Can you work these out from the model? Positions are in its coordinate system, mm. A direction names the side the tool comes from. Round coordinates to 2 decimals unless told otherwise and drop trailing zeros. Order: outer loops, then holes, each group sorted by start corner. A loop starts at its lowest first (then second) coordinate and runs counter-clockwise, first axis right, second up.
Q1. Will this pin go through, and if not, where does the flat tip stop? P1, Ø1, axis at x = -30, y = 16, coming from the -Z side.
Q2. If we section it at D-D (x = 27): Please give me the cut outline in (y, z), plus the area to 3 significant figures.
Q3. If I drill on line 1 (Y direction, x = -27.5, z = 1.7); line 2 (Y direction, x = 36.5, z = 2.05); line 3 (X direction, y = -19.5, z = 0.45), over which ranges is the centre line in solid material (lowest first)?
Q4. We'd pull the mould along Y, two halves only. Please class faces 1 (the face through (42.5, 0, 2)), 2 (the face through (-1, 30, 2)), 3 (the face through (26, 19, 2)): pulls with the +Y half, pulls with the -Y half, needs draft (parallel to the pull), parting line crosses it, or undercut.
Q5. If we section it at C-C (x = -36.5): Please give me the cut outline in (y, z), plus the area to 3 significant figures.
Q6. If we section it at B-B (z = 0.9): Count the separate pieces of the cut face and the enclosed holes in it, plus the area to 3 significant figures.
Q7. For faces 4 (the face through (-32, -20.75, 2)), 5 (the face through (-1, -30, 2)), which set-ups out of +Z, -Z, +X, -X, +Y, -Y let a thin tool reach every point of the face, with its end or its side?
Q8. If we section it at A-A (y = -24.5): Please give me the cut outline in (x, z).
from build123d import *

# Parameters (mm, degrees)
SKETCH1_W              = 85
SKETCH1_H              = 60
SKETCH1_R              = 1.75
SKETCH1_W_2            = 12
SKETCH1_H_2            = 3.5
ELECTRONICS_DECK_DEPTH = 3.2


with BuildPart() as part:
    # Sketch1 → Electronics deck (new body)
    with BuildSketch(Plane.XY):
        Rectangle(SKETCH1_W, SKETCH1_H)
        with Locations((-36.5, -24.5)):
            Circle(SKETCH1_R, mode=Mode.SUBTRACT)
        with Locations((36.5, -24.5)):
            Circle(SKETCH1_R, mode=Mode.SUBTRACT)
        with Locations((-36.5, 24.5)):
            Circle(SKETCH1_R, mode=Mode.SUBTRACT)
        with Locations((36.5, 24.5)):
            Circle(SKETCH1_R, mode=Mode.SUBTRACT)
        with Locations((-32, 19)):
            Rectangle(SKETCH1_W_2, SKETCH1_H_2, mode=Mode.SUBTRACT)
        with Locations((32, 19)):
            Rectangle(SKETCH1_W_2, SKETCH1_H_2, mode=Mode.SUBTRACT)
        with Locations((-32, -19)):
            Rectangle(SKETCH1_W_2, SKETCH1_H_2, mode=Mode.SUBTRACT)
        with Locations((32, -19)):
            Rectangle(SKETCH1_W_2, SKETCH1_H_2, mode=Mode.SUBTRACT)
    extrude(amount=ELECTRONICS_DECK_DEPTH)


solid = part.part
Solution:
1. P1: stops at z = 0
2. outline: (-30, 0) - (-20.75, 0) - (-20.75, 3.2) - (-30, 3.2) - close; (-17.25, 0) - (17.25, 0) - (17.25, 3.2) - (-17.25, 3.2) - close; (20.75, 0) - (30, 0) - (30, 3.2) - (20.75, 3.2) - close
2. area: 170 mm2
3. line 1: y = -30 to -20.75, -17.25 to 17.25, 20.75 to 30
3. line 2: y = -30 to -26.25, -22.75 to -20.75, -17.25 to 17.25, 20.75 to 22.75, 26.25 to 30
3. line 3: x = -42.5 to -38, -26 to 26, 38 to 42.5
4. face 1: needs draft
4. face 2: pulls with the +Y half
4. face 3: undercut
5. outline: (-30, 0) - (-26.25, 0) - (-26.25, 3.2) - (-30, 3.2) - close; (-22.75, 0) - (-20.75, 0) - (-20.75, 3.2) - (-22.75, 3.2) - close; (-17.25, 0) - (17.25, 0) - (17.25, 3.2) - (-17.25, 3.2) - close; (20.75, 0) - (22.75, 0) - (22.75, 3.2) - (20.75, 3.2) - close; (26.25, 0) - (30, 0) - (30, 3.2) - (26.25, 3.2) - close
5. area: 147 mm2
6. separate pieces: 1
6. enclosed holes: 8
6. area: 4,890 mm2
7. face 4: +Z, -Z
7. face 5: +Z, -Z, +X, -X, -Y
8. outline: (-42.5, 0) - (-38.25, 0) - (-38.25, 3.2) - (-42.5, 3.2) - close; (-34.75, 0) - (34.75, 0) - (34.75, 3.2) - (-34.75, 3.2) - close; (38.25, 0) - (42.5, 0) - (42.5, 3.2) - (38.25, 3.2) - close
